Geometry: final body of the model. Coordinates: model frame, mm. A direction names the side the tool comes from. Give positions to 0.01 mm unless a question says otherwise; leave off trailing zeros. Order: outer loops, then holes, each group sorted by start corner. A loop starts at its lowest first (then second) coordinate and runs counter-clockwise, first axis right, second up. Notation, with made-up numbers: (-26.5, -9.75) - (32.5, -9.75) arc R9 ccw to (32.5, 7.25) - close; hole circle Ø11 at (24, 31). An arc over 180 degrees is marked (long way). One line per question, with ' | ' between items. Start each with the question number.
from build123d import *

# Parameters (mm, degrees)
SKETCH1_R               = 1.5
BOSS_EXTRUDE1_DEPTH     = 2.5
SKETCH2_W               = 3.5
SKETCH2_H               = 16
BOSS_EXTRUDE2_DEPTH     = 15
FILLET1_R               = 2
CUT_EXTRUDE1_DEPTH      = 36.889587626
CUT_EXTRUDE1_DEPTH_BACK = 36.889587626
SKETCH3_R               = 3


with BuildPart() as part:
    # Sketch1 → Boss-Extrude1 (new body)
    with BuildSketch(Plane(origin=(0, 0, 0), x_dir=(1, 0, 0), z_dir=(0, 1, 0))):
        with BuildLine():
            Line((15, 20), (-15, 20))
            ThreePointArc((-15, 20), (-18.535533906, 18.535533906), (-20, 15))
            Line((-20, 15), (-20, -15))
            ThreePointArc((-20, -15), (-18.535533906, -18.535533906), (-15, -20))
            Line((-15, -20), (15, -20))
            ThreePointArc((15, -20), (18.535533906, -18.535533906), (20, -15))
            Line((20, -15), (20, 15))
            ThreePointArc((20, 15), (18.535533906, 18.535533906), (15, 20))
        make_face()
        with Locations(Location((10.5, -6.75, 0), (0, 0, 270))):
            Circle(SKETCH1_R, mode=Mode.SUBTRACT)
        with Locations(Location((-10.5, -6.75, 0), (0, 0, 270))):
            Circle(SKETCH1_R, mode=Mode.SUBTRACT)
        with Locations(Location((-10.5, 6.75, 0), (0, 0, 270))):
            Circle(SKETCH1_R, mode=Mode.SUBTRACT)
        with Locations(Location((10.5, 6.75, 0), (0, 0, 270))):
            Circle(SKETCH1_R, mode=Mode.SUBTRACT)
    extrude(amount=BOSS_EXTRUDE1_DEPTH)

    # Sketch2 → Boss-Extrude2 (add)
    with BuildSketch(Plane.XZ):
        with Locations((-4, 0)):
            Rectangle(SKETCH2_W, SKETCH2_H)
        with Locations((4, 0)):
            Rectangle(SKETCH2_W, SKETCH2_H)
    extrude(amount=BOSS_EXTRUDE2_DEPTH)

    # Fillet1
    fillet1_edges = [part.edges().sort_by_distance(p)[0] for p in [
        (-4, -15, -8),
        (-4, -15, 8),
        (4, -15, -8),
        (4, -15, 8),
    ]]
    fillet(fillet1_edges, radius=FILLET1_R)

    # Sketch3 → Cut-Extrude1 (cut, two sides: drawn at the far end of the back side and taken through both)
    with BuildSketch(Plane.ZY.offset(5.75).offset(-CUT_EXTRUDE1_DEPTH_BACK)):
        with Locations((0, -10)):
            Circle(SKETCH3_R)
    extrude(amount=CUT_EXTRUDE1_DEPTH + CUT_EXTRUDE1_DEPTH_BACK, mode=Mode.SUBTRACT)


solid = part.part
(1) Pull-direction query (Z, two-part tool) for faces 4 (the cylindrical face through (-11.41, 1.23, -7.94)), 5 (the cylindrical face through (4.02, -14.4, -7.43)), 6 (the flat face through (-4, -15, 0)); classes: +Z half, -Z half, draft (parallel to the pull), parting line (faces both ways), or undercut.
(2) Cut plane D-D, the plane x = 3. Return the cut outline in (y, z).
(3) Contact query for flat-ended pins moving along their axis: P1, Ø2.5, axis at x = -10.5, z = 6.75, coming from the -Y side; P2, Ø4.5, axis at y = -6.5, z = -2.5, coming from the +X side; P3, Ø1, axis at x = 3.5, y = -5, coming from the +Z side; P4, Ø3, axis at x = 3.5, y = -4.5, coming from the -Z side. Output: stop coordinate, or through.
(4) Cut plane B-B, the plane x = -10.5. Return the cut outline in (y, z), plus the area to 3 significant figures.
(5) Material intervals for line 1 along X through (y, z) = (1, 6.75); line 2 along X through (y, z) = (-2.75, -2); line 3 along Z through (x, y) = (11, 0.75), sorted ascending. Write a range as from..to.
(6) Access query for faces 1 (the flat face through (-4, -6, -8)), 2 (the flat face through (-4, -6, 8)), 3 (the flat face through (2.25, -6, 0)). Directions: +Z, -Z, +X, -X, +Y, -Y. A direction counts if a zero-diameter tool reaches every point of the face in a straight line with its end or side. Return the directions, or none.
(7) Cut plane C-C, the plane y = -6. Return the cut outline in (x, z).
(8) Cut plane A-A, the plane y = -10. Return the cut outline in (x, z).
Results are:
1) face 4: undercut | face 5: -Z half | face 6: draft
2) outline: (-15, -6) arc R2 ccw to (-13, -8) - (0, -8) - (0, -20) - (2.5, -20) - (2.5, 20) - (0, 20) - (0, 8) - (-13, 8) arc R2 ccw to (-15, 6) - close; hole circle Ø6 at (-10, 0)
3) P1: through | P2: x = 5.75 | P3: z = 8 | P4: z = -8
4) outline: (0, -20) - (2.5, -20) - (2.5, -8.25) - (0, -8.25) - close; (0, -5.25) - (2.5, -5.25) - (2.5, 5.25) - (0, 5.25) - close; (0, 8.25) - (2.5, 8.25) - (2.5, 20) - (0, 20) - close | area: 85.0 mm2
5) line 1: -20..-12, -9..9, 12..20 | line 2: -5.75..-2.25, 2.25..5.75 | line 3: -20..-8.16, -5.34..5.34, 8.16..20
6) face 1: -Z, +X, -X, -Y | face 2: +Z, +X, -X, -Y | face 3: +Z, -Z, -Y
7) outline: (-5.75, -8) - (-2.25, -8) - (-2.25, 8) - (-5.75, 8) - close; (2.25, -8) - (5.75, -8) - (5.75, 8) - (2.25, 8) - close
8) outline: (-5.75, -8) - (-2.25, -8) - (-2.25, -3) - (-5.75, -3) - close; (-5.75, 3) - (-2.25, 3) - (-2.25, 8) - (-5.75, 8) - close; (2.25, -8) - (5.75, -8) - (5.75, -3) - (2.25, -3) - close; (2.25, 3) - (5.75, 3) - (5.75, 8) - (2.25, 8) - close
